Build history of the part. All positions in model axes, mm. Round coordinates to 2 decimals unless told otherwise and drop trailing zeros. Loops run counter-clockwise (first coordinate to the right, second up) from the corner with the lowest first, then second, coordinate; pieces in that order, holes last. Notation, with made-up numbers: (59, 77) - (64, 77) arc R34 ccw to (64, 113) - close; hole circle Ø11 at (26.25, 3). An arc over 180 degrees is marked (long way). Use a Markdown table: item, result.
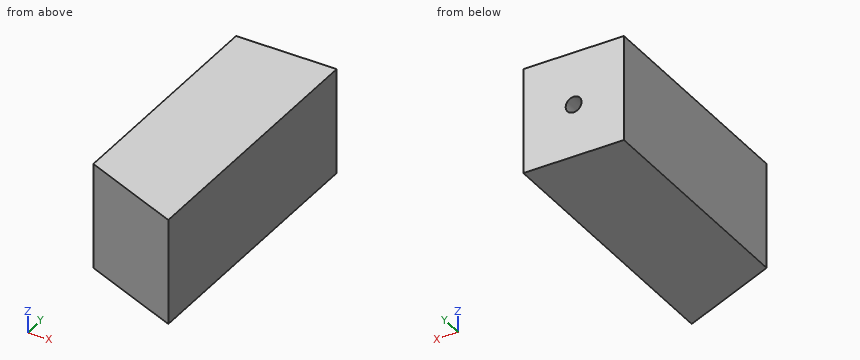
from build123d import *

# Parameters (mm, degrees)
EXTRUDE_1_DEPTH     = 20
SKETCH_2_R          = 1.5
CUT_EXTRUDE_1_DEPTH = 20


with BuildPart() as part:
    # 草图1 → 凸台-拉伸1 (new body)
    with BuildSketch(Plane.XY):
        Polygon((10.5, 12), (29.5, 4), (29.5, 56.5), (10.5, 56.5), align=None)
    extrude(amount=-EXTRUDE_1_DEPTH)

    # 草图2 → 切除-拉伸1 (cut)
    with BuildSketch(Plane(origin=(0, 56.5, 0), x_dir=(1, 0, 0), z_dir=(0, 1, 0))):
        with Locations(Location((20, 10, 0), (0, 0, 270))):
            Circle(SKETCH_2_R)
    extrude(amount=-CUT_EXTRUDE_1_DEPTH, mode=Mode.SUBTRACT)


solid = part.part
Q1. Cut at A-A, the plane y = 49. List the corners of the cut face in (x, z).
Results found:
| item | result |
|---|---|
| outline | (10.5, -20) - (29.5, -20) - (29.5, 0) - (10.5, 0) - close; hole circle Ø3 at (20, -10) |
Q2. Cut at B-B, the plane z = -10. List the corners of the cut face in (x, y).
Results found:
| item | result |
|---|---|
| outline | (10.5, 12) - (29.5, 4) - (29.5, 56.5) - (21.5, 56.5) - (21.5, 36.5) - (18.5, 36.5) - (18.5, 56.5) - (10.5, 56.5) - close |
Q3. Probe line 1 (X direction, y = 42, z = -10); line 2 (Z direction, x = 21, y = 52); line 3 (Y direction, x = 18.5, z = -6). List the from-to ranges inside material, lowest first.
Results found:
| item | result |
|---|---|
| line 1 | x = 10.5 to 18.5, 21.5 to 29.5 |
| line 2 | z = -20 to -11.12, -8.88 to 0 |
| line 3 | y = 8.63 to 56.5 |
Q4. Cut at D-D, the plane z = -15.25. List the corners of the cut face in (x, y).
Results found:
| item | result |
|---|---|
| outline | (10.5, 12) - (29.5, 4) - (29.5, 56.5) - (10.5, 56.5) - close |
Q5. Drop flat-ended pins along their axis: pin 1 (1 mm diameter, centred on x = 13, z = -17, fed in from -Y); pin 2 (0.9 mm diameter, centred on x = 20, z = -10, fed in from +Y); pin 3 (2.5 mm diameter, centred on x = 20, z = -10, fed in from -Y). Give the stop position or say it passes through.
Results found:
| item | result |
|---|---|
| pin 1 | stops at y = 10.74 |
| pin 2 | stops at y = 36.5 |
| pin 3 | stops at y = 7.47 |
Q6. Cut at C-C, the plane x = 24.75. List the corners of the cut face in (y, z).
Results found:
| item | result |
|---|---|
| outline | (6, -20) - (56.5, -20) - (56.5, 0) - (6, 0) - close |
